Here's how the part is built. I have some questions about the finished solid (model axes, mm). Round coordinates to 2 decimals unless told otherwise and drop trailing zeros. Write each loop counter-clockwise with the first axis right and the second up, starting at its lowest first coordinate (ties: lowest second). Pieces come first, ordered by that corner, then holes. Notation, with made-up numbers: (4, 25) - (50, 25) arc R20 cw to (50, 33) - close; hole circle Ø3 at (49.5, 26). An arc over 180 degrees is marked (long way). One line per item, written item: value. Start each with the question number.
Item 1: Imagine slicing it at B-B, the plane z = -170. Please give me the cut outline in (x, y).
Item 2: Imagine slicing it at A-A, the plane x = -66.5. Please give me the cut outline in (y, z), then the cut area to 3 significant figures.
Item 3: Imagine slicing it at D-D, the plane x = -11.5. Please give me the cut outline in (y, z).
Item 4: If I drill on line 1 (X direction, y = 1, z = -31); line 2 (Z direction, x = -113.5, y = 7.5); line 3 (X direction, y = 5.5, z = -173), over which ranges is the centre line in solid material (lowest first)?
Item 5: Imagine slicing it at C-C, the plane y = 2.75. Count the separate pieces of the cut face and the enclosed holes in it, then the cut area to 3 significant figures.
Item 6: For P1, Ø6, axis at x = -150, z = -207, coming from the +Y side; P2, Ø5, axis at x = -24, y = 6.5, coming from the +Z side; P3, Ø1.5, axis at y = 4, z = -235, coming from the +X side; P4, Ø3, axis at x = -21.5, y = 2.5, coming from the -Z side, each with a flat end and sliding along its axis, tell me the tip position at first contact or that it passes through.
```python
from build123d import *

# Parameters (mm, degrees)
SKETCH1_W           = 14.703470952
SKETCH1_H           = 200.333333333
SKETCH1_W_2         = 57.995054435
SKETCH1_H_2         = 47.634748305
BOSS_EXTRUDE1_DEPTH = 10


with BuildPart() as part:
    # Sketch1 → Boss-Extrude1 (new body)
    with BuildSketch(Plane(origin=(0, 0, 0), x_dir=(1, 0, 0), z_dir=(0, 1, 0))):
        with BuildLine():
            Line((0, 5), (0, 209.09430585))
            ThreePointArc((0, 209.09430585), (-0.25658351, 210.67544468), (-1, 212.09430585))
            Line((-1, 212.09430585), (-32.74341649, 254.41886117))
            ThreePointArc((-32.74341649, 254.41886117), (-33.17231305, 255.098327769), (-33.486832981, 255.83772234))
            Line((-33.486832981, 255.83772234), (-49.298221281, 303.271887242))
            ThreePointArc((-49.298221281, 303.271887242), (-51.118086348, 305.746959338), (-54.041637772, 306.690748412))
            Line((-54.041637772, 306.690748412), (-118.887294417, 306.690748412))
            ThreePointArc((-118.887294417, 306.690748412), (-121.81084584, 305.746959338), (-123.630710907, 303.271887242))
            Line((-123.630710907, 303.271887242), (-139.442099208, 255.83772234))
            ThreePointArc((-139.442099208, 255.83772234), (-139.756619138, 255.098327769), (-140.185515698, 254.41886117))
            Line((-140.185515698, 254.41886117), (-171.928932188, 212.09430585))
            ThreePointArc((-171.928932188, 212.09430585), (-172.672348678, 210.67544468), (-172.928932188, 209.09430585))
            Line((-172.928932188, 209.09430585), (-172.928932188, 5))
            ThreePointArc((-172.928932188, 5), (-171.464466094, 1.464466094), (-167.928932188, 0))
            Line((-167.928932188, 0), (-147.071067812, 0))
            ThreePointArc((-147.071067812, 0), (-145.15765065, -0.380602337), (-143.535533906, -1.464466094))
            Line((-143.535533906, -1.464466094), (-117.928932188, -27.071067812))
            ThreePointArc((-117.928932188, -27.071067812), (-116.306815444, -28.154931568), (-114.393398282, -28.535533906))
            Line((-114.393398282, -28.535533906), (-58.535533906, -28.535533906))
            ThreePointArc((-58.535533906, -28.535533906), (-56.622116744, -28.154931568), (-55, -27.071067812))
            Line((-55, -27.071067812), (-29.393398282, -1.464466094))
            ThreePointArc((-29.393398282, -1.464466094), (-27.771281538, -0.380602337), (-25.857864376, 0))
            Line((-25.857864376, 0), (-5, 0))
            ThreePointArc((-5, 0), (-1.464466094, 1.464466094), (0, 5))
        make_face()
        with Locations((-22.648264524, 110.59430585)):
            Rectangle(SKETCH1_W, SKETCH1_H, mode=Mode.SUBTRACT)
        with Locations((-150.280667664, 110.59430585)):
            Rectangle(SKETCH1_W, SKETCH1_H, mode=Mode.SUBTRACT)
        with Locations((-86.464466095, 178.682625847)):
            Rectangle(SKETCH1_W_2, SKETCH1_H_2, mode=Mode.SUBTRACT)
    extrude(amount=BOSS_EXTRUDE1_DEPTH)


solid = part.part
```
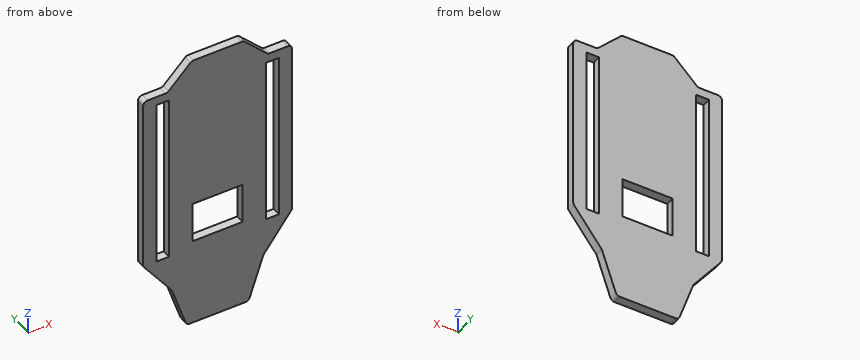
Values follow:
1. outline: (-172.93, 0) - (-157.63, 0) - (-157.63, 10) - (-172.93, 10) - close; (-142.93, 0) - (-115.46, 0) - (-115.46, 10) - (-142.93, 10) - close; (-57.47, 0) - (-30, 0) - (-30, 10) - (-57.47, 10) - close; (-15.3, 0) - (0, 0) - (0, 10) - (-15.3, 10) - close
2. outline: (0, -306.69) - (10, -306.69) - (10, -202.5) - (0, -202.5) - close; (0, -154.87) - (10, -154.87) - (10, 28.54) - (0, 28.54) - close
2. area: 2,880 mm^2
3. outline: (0, -226.09) - (10, -226.09) - (10, 0) - (0, 0) - close
4. line 1: x = -172.93 to -157.63, -142.93 to -30, -15.3 to 0
4. line 2: z = -306.69 to -202.5, -154.87 to 28.54
4. line 3: x = -172.93 to -157.63, -142.93 to -115.46, -57.47 to -30, -15.3 to 0
5. separate pieces: 1
5. enclosed holes: 3
5. area: 41,100 mm^2
6. P1: passes through
6. P2: stops at z = 0.04
6. P3: stops at x = -17.62
6. P4: stops at z = -241.43
